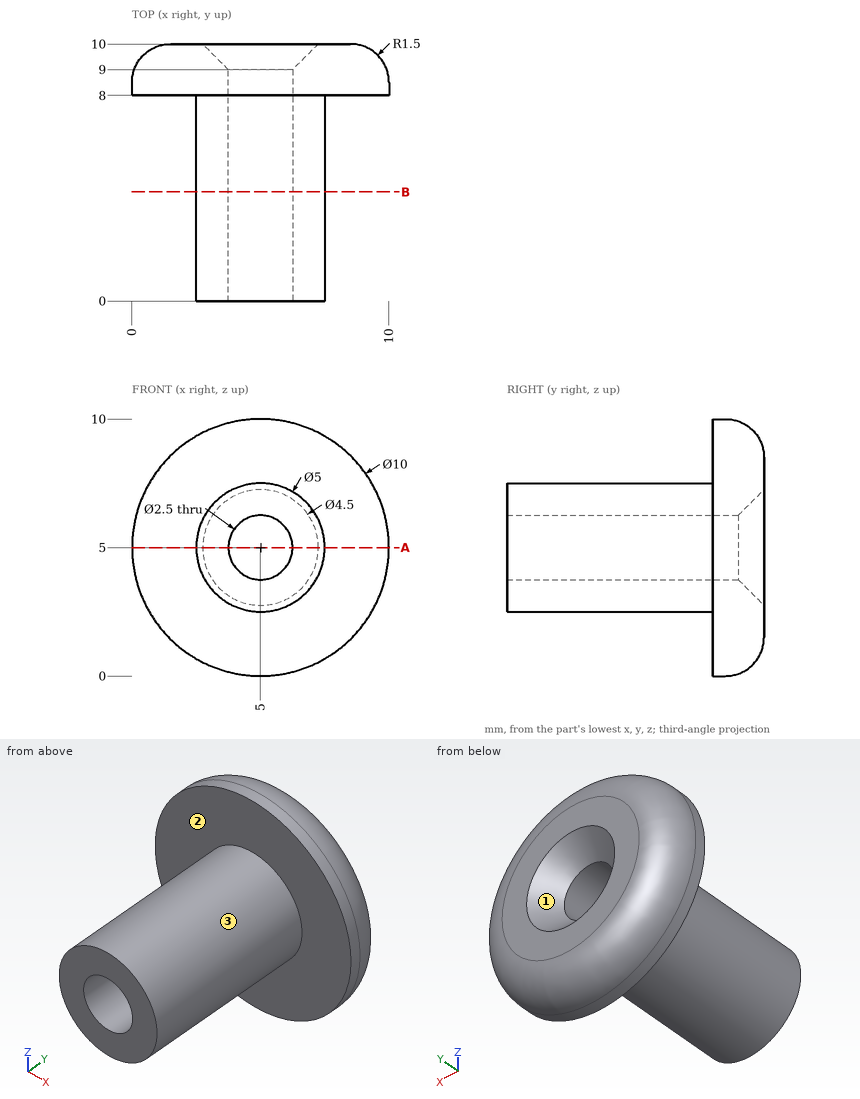
Study the drawing (mm; zero at the part's minimum x, y, z) and answer. Coordinates: 2 decimals unless noted, no trailing zeros. Write each loop counter-clockwise with the first axis right and the second up, starting at its lowest first coordinate (ties: lowest second). Pieces come first, ordered by that corner, then holes. Notation, with made-up numbers: (67.25, 31) - (87.25, 31) arc R22 cw to (87.25, 55) - close; hole circle Ø10 at (21.5, 58). An arc over 180 degrees is marked (long way). Answer as a JSON object with one key per item and string values.
Q1. Consider L1, parallel to Z at x = 5, y = 3.5; L2, parallel to X at y = 9.25, z = 4.25; L3, parallel to Z at x = 4.25, y = 6.5. Determine where each line is inside the solid, lowest interval first. Write a range as from..to.
Results list:
{"L1": "z = 2.5..3.75, 6.25..7.5", "L2": "x = 0.26..3.7, 6.3..9.74", "L3": "z = 2.62..4, 6..7.38"}
Q2. Given pin 1 Ø3 at (x, z) = (3.5, 3.5) entering from -Y; pin 2 Ø1 at (y, z) = (3, 4.5) entering from -X, each flat-ended and moving along its own axis, determine where each tip first touches the part or whether it passes through.
Results list:
{"pin 1": "stops at y = 0", "pin 2": "stops at x = 2.5"}
Q3. For a pull along Z with two mould halves and no side action, classify the marked faces 1, 2 and 3 as pulls with the +Z half, pulls with the -Z half, needs draft (parallel to the pull), parting line crosses it, or undercut.
Results list:
{"face 1": "undercut", "face 2": "needs draft", "face 3": "parting line crosses it"}
Q4. Find section A-A (z = 5). Write down the section's boundary in (x, y), plus the area to 3 significant figures.
Results list:
{"outline": "(0, 8) - (2.5, 8) - (2.5, 0) - (3.75, 0) - (3.75, 9) - (2.75, 10) - (1.5, 10) arc R1.5 ccw to (0, 8.5) - close; (6.25, 0) - (7.5, 0) - (7.5, 8) - (10, 8) - (10, 8.5) arc R1.5 ccw to (8.5, 10) - (7.25, 10) - (6.25, 9) - close", "area": "33.0 mm^2"}
Q5. Find section B-B (y = 4.25). Write down the section's boundary in (x, z).
Results list:
{"outline": "circle Ø5 at (5, 5); hole circle Ø2.5 at (5, 5)"}
